from build123d import *

# Parameters (mm, degrees)
EXTRUDE_1_DEPTH     = 5
EXTRUDE_2_DEPTH     = 1
SKETCH_3_R          = 6
EXTRUDE_3_DEPTH     = 3
SKETCH_4_R          = 3
EXTRUDE_4_DEPTH     = 1.5
SKETCH_6_W          = 4
SKETCH_6_H          = 6
EXTRUDE_5_DEPTH     = 2.5
SKETCH_7_R          = 1
CUT_EXTRUDE_1_DEPTH = 5


with BuildPart() as part:
    # Эскиз1 → Бобышка-Вытянуть1 (new body)
    with BuildSketch(Plane(origin=(0, 0, 0), x_dir=(1, 0, 0), z_dir=(0, 1, 0))):
        Polygon((-29.797958971, -5), (-29.797958971, 5), (-20.578414514, 11), (19.421585486, 11), (27.5, 7.5), (27.5, -6), (20, -10), (-20, -10), align=None)
    extrude(amount=EXTRUDE_1_DEPTH)

    # Эскиз2 → Бобышка-Вытянуть2 (add)
    with BuildSketch(Plane(origin=(0, 5, 0), x_dir=(1, 0, 0), z_dir=(0, 1, 0))):
        with BuildLine():
            Line((-23.797958971, 7.5), (-18.530009779, 7.5))
            ThreePointArc((-18.530009779, 7.5), (-16.797958971, 10.5), (-15.065908164, 7.5))
            Line((-15.065908164, 7.5), (-9.797958971, 7.5))
            Line((-9.797958971, 7.5), (-9.797958971, -6.5))
            Line((-9.797958971, -6.5), (-15.065908164, -6.5))
            ThreePointArc((-15.065908164, -6.5), (-16.797958971, -9.5), (-18.530009779, -6.5))
            Line((-18.530009779, -6.5), (-23.797958971, -6.5))
            Line((-23.797958971, -6.5), (-23.797958971, 7.5))
        make_face()
    extrude(amount=EXTRUDE_2_DEPTH)

    # Эскиз3 → Бобышка-Вытянуть3 (add)
    with BuildSketch(Plane(origin=(0, 6, 0), x_dir=(1, 0, 0), z_dir=(0, 1, 0))):
        with Locations(Location((-16.797958971, 0.5, 0), (0, 0, 270))):
            Circle(SKETCH_3_R)
    extrude(amount=EXTRUDE_3_DEPTH)

    # Эскиз4 → Бобышка-Вытянуть4 (add)
    with BuildSketch(Plane(origin=(0, 5, 0), x_dir=(1, 0, 0), z_dir=(0, 1, 0))):
        with Locations(Location((-0.797958971, 0.5, 0), (0, 0, 90))):
            Circle(SKETCH_4_R)
    extrude(amount=EXTRUDE_4_DEPTH)

    # Эскиз6 → Бобышка-Вытянуть5 (add)
    with BuildSketch(Plane.XZ):
        with Locations((17.5, 5.5)):
            Rectangle(SKETCH_6_W, SKETCH_6_H)
    extrude(amount=EXTRUDE_5_DEPTH)

    # Эскиз7 → Вырез-Вытянуть1 (cut)
    with BuildSketch(Plane(origin=(0, 5, 0), x_dir=(1, 0, 0), z_dir=(0, 1, 0))):
        with Locations(Location((-26.047958971, -5.25, 0), (0, 0, 270))):
            Circle(SKETCH_7_R)
        with Locations(Location((25.5, 6.5, 0), (0, 0, 270))):
            Circle(SKETCH_7_R)
    extrude(amount=-CUT_EXTRUDE_1_DEPTH, mode=Mode.SUBTRACT)


solid = part.part
The listing builds one solid part. Answer for the finished solid, in the listing's coordinates (mm). A direction names the side the tool comes from. Coordinates: 2 decimals unless noted, no trailing zeros. Loops run counter-clockwise (first coordinate to the right, second up) from the corner with the lowest first, then second, coordinate; pieces in that order, holes last. Notation, with made-up numbers: (19, 31) -> (43, 31) arc R21 ccw to (43, 70) -> close; hole circle Ø8 at (-40, -38.5). An arc over 180 degrees is marked (long way). Answer in a Markdown table with one row per item. Add a question column.
1. The part is cut by section C-C, the plane x = 25.5. Write down the section's boundary in (y, z), then the cut area to 3 significant figures.
2. Determine the mould class of faces 6 (the flat face through (23.404, 2.465, -9.274)), 7 (the cylindrical face through (-16.74, 5.49, 9.5)), 8 (the flat face through (6, 5, -1)) for opening direction Z: +Z half, -Z half, draft (parallel to the pull), parting line (faces both ways), or undercut.
3. The part is cut by section D-D, the plane y = -0.5. Write down the section's boundary in (x, z), then the cut area to 3 significant figures.
4. The part is cut by section B-B, the plane z = -0.5. Write down the section's boundary in (x, y).
5. Flat-ended cylindrical pins translate along their axes: P1, Ø3, axis at x = -2, z = -0.5, coming from the +Y side; P2, Ø2, axis at x = 5, z = 3.5, coming from the +Y side; P3, Ø0.8, axis at x = -13, y = 5.5, coming from the -Z side. Find the tip coordinate at first contact, or state that the pin passes through.
6. For faces 1 (the flat face through (19.5, -1, 5)), 2 (the flat face through (-9.798, 5.5, -0.6)), 3 (the flat face through (15.5, -1, 5)), 4 (the flat face through (-10, 6, -1)), 5 (the flat face through (-1, 6.5, 0)), determine the directions among +Z, -Z, +X, -X, +Y, -Y from which every point of the face is accessible in a straight line to the end or side of a thin tool.
7. Consider line 1 (Y direction, x = 16, z = -10); line 2 (X direction, y = 3.85, z = -6.5); line 3 (X direction, y = 3.5, z = 5.25). Determine where each line is inside the solid, lowest interval first. Write a range as [from, to].
8. The part is cut by section A-A, the plane y = 3. Write down the section's boundary in (x, z).
Answer below:
| question | item | result |
|---|---|---|
| 1 | outline | (0, -8.37) -> (5, -8.37) -> (5, -7.5) -> (0, -7.5) -> close; (0, -5.5) -> (5, -5.5) -> (5, 7.07) -> (0, 7.07) -> close |
| 1 | area | 67.2 mm2 |
| 2 | face 6 | -Z half |
| 2 | face 7 | undercut |
| 2 | face 8 | draft |
| 3 | outline | (15.5, 2.5) -> (19.5, 2.5) -> (19.5, 8.5) -> (15.5, 8.5) -> close |
| 3 | area | 24.0 mm2 |
| 4 | outline | (-29.8, 0) -> (27.5, 0) -> (27.5, 5) -> (2.2, 5) -> (2.2, 6.5) -> (-3.8, 6.5) -> (-3.8, 5) -> (-9.8, 5) -> (-9.8, 6) -> (-10.8, 6) -> (-10.8, 9) -> (-22.8, 9) -> (-22.8, 6) -> (-23.8, 6) -> (-23.8, 5) -> (-29.8, 5) -> close |
| 5 | P1 | y = 6.5 |
| 5 | P2 | y = 5 |
| 5 | P3 | z = -7.5 |
| 6 | face 1 | +Z, -Z, +X, -Y |
| 6 | face 2 | +Z, -Z, +Y |
| 6 | face 3 | +Z, -Z, -X, -Y |
| 6 | face 4 | +Y |
| 6 | face 5 | +Z, -Z, +X, +Y |
| 7 | line 1 | [0, 5] |
| 7 | line 2 | [-27.49, 24.5], [26.5, 27.5] |
| 7 | line 3 | [-29.31, -27.05], [-25.05, 27.5] |
| 8 | outline | (-29.8, -5) -> (-20.58, -11) -> (19.42, -11) -> (27.5, -7.5) -> (27.5, 6) -> (20, 10) -> (-20, 10) -> (-29.8, 5) -> close; hole circle Ø2 at (-26.05, 5.25); hole circle Ø2 at (25.5, -6.5) |
